Can you work these out from the model? Positions are in its coordinate system, mm. Face numbers are marked on the shaded views. Round coordinates to 2 decimals unless told otherwise and drop trailing zeros. Write each loop counter-clockwise with the first axis right and the second up, starting at its lowest first coordinate (ties: lowest second). Pieces come first, ordered by that corner, then holes. Notation, with made-up numbers: M 88,75 L 119,75 A22 cw 119,106 Z; hole C 69,5.25 d2. An arc over 180 degrees is marked long. Use one line per item in the form item = value. Start each with the question number.
```python
from build123d import *

# Parameters (mm, degrees)
SKETCH1_W                        = 160.02
SKETCH1_H                        = 127
BOSS_EXTRUDE1_DEPTH              = 6.35
FILLET1_R                        = 2.54
SHELL1_START                     = 2.54
SHELL1_OUTLINE_W                 = 121.92
SHELL1_OUTLINE_H                 = 3.81
SHELL1_DEPTH                     = 154.94
CHAMFER1_SIZE                    = 10.16
F_9_64_0_15_DIAMETER_HOLE1_D     = 3.81
F_9_64_0_15_DIAMETER_HOLE1_DEPTH = 6.35
F_9_64_0_15_DIAMETER_HOLE1_TIP   = 1.144639479


# Read off the part's stored shape, not the designer's step: Shell1
with BuildPart() as part:
    # Sketch1 → Boss-Extrude1 (new body)
    with BuildSketch(Plane.XY):
        with Locations((80.01, -63.5)):
            Rectangle(SKETCH1_W, SKETCH1_H)
    extrude(amount=BOSS_EXTRUDE1_DEPTH)

    # Fillet1
    fillet1_edges = [part.edges().sort_by_distance(p)[0] for p in [
        (160.02, -63.5, 6.35),
        (80.01, 0, 6.35),
        (0, -63.5, 6.35),
        (0, 0, 3.175),
        (160.02, 0, 3.175),
        (160.02, -127, 3.175),
        (0, -127, 3.175),
        (80.01, -127, 6.35),
    ]]
    fillet(fillet1_edges, radius=FILLET1_R)

    # Shell1 outline → Shell1 (cut)
    with BuildSketch(Plane.YZ.offset(SHELL1_START)):
        with Locations((-63.5, 1.905)):
            Rectangle(SHELL1_OUTLINE_W, SHELL1_OUTLINE_H)
    extrude(amount=SHELL1_DEPTH, mode=Mode.SUBTRACT)

    # Chamfer1
    chamfer1_edges = [part.edges().sort_by_distance(p)[0] for p in [
        (2.54, -2.54, 1.905),
        (2.54, -124.46, 1.905),
        (157.48, -124.46, 1.905),
        (157.48, -2.54, 1.905),
    ]]
    chamfer(chamfer1_edges, length=CHAMFER1_SIZE)

    # 9/64 (0.15) Diameter Hole1
    with Locations(Plane(origin=(0, 0, 0), x_dir=(-1, 0, 0), z_dir=(0, 0, -1))):
        with Locations((-155.2575, -4.7625), (-4.7625, -4.7625), (-4.7625, -122.2375), (-155.2575, -122.2375)):
            Hole(F_9_64_0_15_DIAMETER_HOLE1_D / 2, depth=F_9_64_0_15_DIAMETER_HOLE1_DEPTH)
            with Locations((0, 0, -(F_9_64_0_15_DIAMETER_HOLE1_DEPTH + F_9_64_0_15_DIAMETER_HOLE1_TIP / 2))):  # 118° drill point
                Cone(0, F_9_64_0_15_DIAMETER_HOLE1_D / 2, F_9_64_0_15_DIAMETER_HOLE1_TIP, mode=Mode.SUBTRACT)


solid = part.part
```
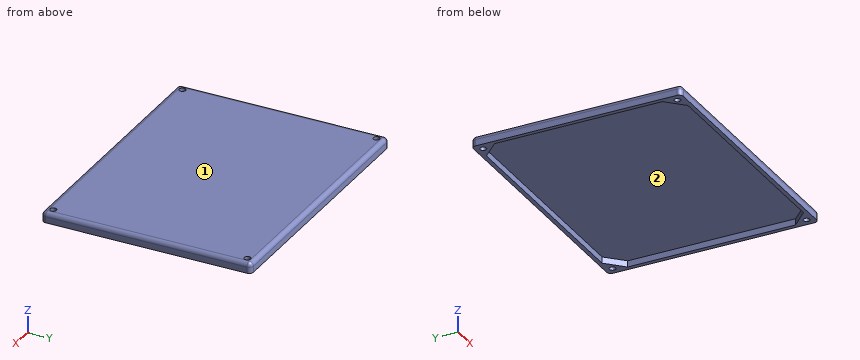
1. If we mould it in two halves opening along Z, with no side actions, what happens to the marked faces 1 and 2? For each: pulls with the +Z half, pulls with the -Z half, needs draft (parallel to the pull), parting line crosses it, or undercut.
2. If we section it at B-B (z = 1): List the corners of the cut face in (x, y) for me (1 decimal), and give its area (3 significant figures).
3. Will these pins go through, and if not, where does the flat tip stop? pin 1 (5 mm diameter, centred on x = 141.5, y = -98.5, fed in from -Z); pin 2 (1 mm diameter, centred on x = 123, z = 5, fed in from -Y); pin 3 (1 mm diameter, centred on y = -29, z = 5.5, fed in from +X).
4. If we section it at C-C (y = -19.5): List the corners of the cut face in (x, z) for me.
5. If we section it at A-A (x = 150): List the corners of the cut face in (y, z) for me.
6. Please list where these lines run through material, in increasing order: line 1 along Y through (x, z) = (46, 0.75); line 2 along X through (y, z) = (-48.5, 0.75); line 3 along Z through (x, y) = (99, -22.5).
Model answer:
q1.face_1 = pulls with the +Z half
q1.face_2 = pulls with the -Z half
q2.outline = M 0,-124.5 A2.5 ccw 2.5,-127 L 157.5,-127 A2.5 ccw 160,-124.5 L 160,-2.5 A2.5 ccw 157.5,0 L 2.5,0 A2.5 ccw 0,-2.5 Z; hole M 2.5,-114.3 L 12.7,-124.5 L 147.3,-124.5 L 157.5,-114.3 L 157.5,-12.7 L 147.3,-2.5 L 12.7,-2.5 L 2.5,-12.7 Z; hole C 4.8,-122.2 d3.8; hole C 4.8,-4.8 d3.8; hole C 155.3,-122.2 d3.8; hole C 155.3,-4.8 d3.8
q2.area = 1,590 mm2
q3.pin_1 = 3.81
q3.pin_2 = -126.9
q3.pin_3 = 159.72
q4.outline = M 0,0 L 2.54,0 L 2.54,3.81 L 157.48,3.81 L 157.48,0 L 160.02,0 L 160.02,3.81 A2.54 ccw 157.48,6.35 L 2.54,6.35 A2.54 ccw 0,3.81 Z
q5.outline = M -127,0 L -121.78,0 L -121.78,3.81 L -5.22,3.81 L -5.22,0 L 0,0 L 0,3.81 A2.54 ccw -2.54,6.35 L -124.46,6.35 A2.54 ccw -127,3.81 Z
q6.line_1 = -127 to -124.46, -2.54 to 0
q6.line_2 = 0 to 2.54, 157.48 to 160.02
q6.line_3 = 3.81 to 6.35
